from build123d import *

# Parameters (mm, degrees)
F0_R     = 1.5
F0_R_2   = 1.75
F1_DEPTH = 7
F2_R     = 2.5
F2_R_2   = 1.75
F2_R_3   = 2.25
F2_R_4   = 1.5
F3_DEPTH = 3
F5_DEPTH = 25


with BuildPart() as f1:
    # F0 (on Top) → F1 (new body)
    with BuildSketch(Plane.XY):
        Polygon((22.5, 0), (22.5, 5), (-22.5, 5), (-22.5, 0), (-22.5, -5), (22.5, -5), align=None)
        with BuildLine():
            ThreePointArc((-15.75, 0), (-17.5, -1.75), (-19.25, 0))
            ThreePointArc((-19.25, 0), (-17.5, 1.75), (-15.75, 0))
        make_face(mode=Mode.SUBTRACT)
        with Locations((-4.5, 0)):
            Circle(F0_R, mode=Mode.SUBTRACT)
        with Locations((4.5, 0)):
            Circle(F0_R, mode=Mode.SUBTRACT)
        with Locations((17.5, 0)):
            Circle(F0_R_2, mode=Mode.SUBTRACT)
    extrude(amount=F1_DEPTH)

    # F2 (on face) → F3 (cut)
    with BuildSketch(Plane.XY.offset(7)):
        with Locations((-17.5, 0)):
            Circle(F2_R)
        with Locations((-17.5, 0)):
            Circle(F2_R_2, mode=Mode.SUBTRACT)
        with Locations((-4.5, 0)):
            Circle(F2_R_3)
        with Locations((-4.5, 0)):
            Circle(F2_R_4, mode=Mode.SUBTRACT)
        with Locations((4.5, 0)):
            Circle(F2_R_3)
        with Locations((4.5, 0)):
            Circle(F2_R_4, mode=Mode.SUBTRACT)
        with Locations((17.5, 0)):
            Circle(F2_R)
        with Locations((17.5, 0)):
            Circle(F2_R_2, mode=Mode.SUBTRACT)
    extrude(amount=-F3_DEPTH, mode=Mode.SUBTRACT)

    # F4 (on face) → F5 (cut)
    with BuildSketch(Plane(origin=(0, 5, 0), x_dir=(-1, 0, 0), z_dir=(0, 1, 0))):
        with BuildLine():
            Line((0, 7), (-7.72596329, 7))
            ThreePointArc((-7.72596329, 7), (0, 3.3733951654), (7.72596329, 7))
            Line((7.72596329, 7), (0, 7))
        make_face()
    extrude(amount=-F5_DEPTH, mode=Mode.SUBTRACT)


solid = f1.part
Work out the finished part from the listing and answer in its coordinate system (mm). A direction names the side the tool comes from. Give positions to 0.01 mm unless a question says otherwise; leave off trailing zeros. Order: outer loops, then holes, each group sorted by start corner. A loop starts at its lowest first (then second) coordinate and runs counter-clockwise, first axis right, second up. Notation, with made-up numbers: (54.25, 39) -> (105.25, 39) arc R14 ccw to (105.25, 54) -> close; hole circle Ø7 at (-18, -33.75). An arc over 180 degrees is marked (long way). One line per item, written item: value.
Item 1: Flat-ended cylindrical pins translate along their axes: P1, Ø3, axis at x = -11, y = 0, coming from the -Z side; P2, Ø3, axis at x = 3.5, y = -1, coming from the +Z side; P3, Ø1, axis at x = -5.5, y = -1, coming from the +Z side. Find the tip coordinate at first contact, or state that the pin passes through.
Answer sheet:
P1: z = 0
P2: z = 4.36
P3: z = 4
Item 2: Straight lines are drawn through the part: probe 1 along Y at (x, z) = (4.5, 2.1); probe 2 along X at (y, z) = (1, 5); probe 3 along Y at (x, z) = (17.5, 5.25). For each, find the intervals that lie inside material, in ascending order.
Answer sheet:
probe 1: -5 to -1.5, 1.5 to 5
probe 2: -22.5 to -19.79, -15.21 to -6.52, 6.52 to 15.21, 19.79 to 22.5
probe 3: -5 to -2.5, 2.5 to 5
Item 3: Find section C-C, the plane z = 5. Give the vertices of the cut face in (x, y), plus the area to 3 significant figures.
Answer sheet:
outline: (-22.5, -5) -> (-5.48, -5) -> (-5.48, -2.03) arc R2.25 cw to (-5.48, 2.03) -> (-5.48, 5) -> (-22.5, 5) -> close; (5.48, -5) -> (22.5, -5) -> (22.5, 5) -> (5.48, 5) -> (5.48, 2.03) arc R2.25 cw to (5.48, -2.03) -> close; hole circle Ø5 at (-17.5, 0); hole circle Ø5 at (17.5, 0)
area: 294 mm²
Item 4: Find section D-D, the plane z = 0.5. Give the vertices of the cut face in (x, y), plus the area to 3 significant figures.
Answer sheet:
outline: (-22.5, -5) -> (22.5, -5) -> (22.5, 5) -> (-22.5, 5) -> close; hole circle Ø3.5 at (-17.5, 0); hole circle Ø3 at (-4.5, 0); hole circle Ø3 at (4.5, 0); hole circle Ø3.5 at (17.5, 0)
area: 417 mm²
Item 5: Find section A-A, the plane x = -17.5. Give the vertices of the cut face in (y, z).
Answer sheet:
outline: (-5, 0) -> (-1.75, 0) -> (-1.75, 4) -> (-2.5, 4) -> (-2.5, 7) -> (-5, 7) -> close; (1.75, 0) -> (5, 0) -> (5, 7) -> (2.5, 7) -> (2.5, 4) -> (1.75, 4) -> close
Item 6: Find section B-B, the plane y = 0. State how many separate pieces and enclosed holes the cut face has, plus the area to 3 significant figures.
Answer sheet:
separate pieces: 5
enclosed holes: 0
area: 189 mm²
Item 7: A tool of negligible diameter and unlimited length cuts with its end or side. For faces 1 (the cylindrical face through (0.123, 0.07, 3.374)), 2 (the cylindrical face through (-6.75, 0.06, 4.79)), from which of +Z, -Z, +X, -X, +Y, -Y can it reach the whole face along a straight path? Write none if from no direction.
Answer sheet:
face 1: +Z, +Y, -Y
face 2: +Z
